Design review of the part built by this model. Coordinates are the model's own, in mm. A direction names the side the tool comes from. Round coordinates to 2 decimals unless told otherwise and drop trailing zeros. Order: outer loops, then holes, each group sorted by start corner. A loop starts at its lowest first (then second) coordinate and runs counter-clockwise, first axis right, second up. Notation, with made-up numbers: (-12, -16) - (45, -16) arc R19 cw to (45, 12) - close; hole circle Ø7 at (-38, 64.5). An arc over 180 degrees is marked (long way). Use CSV: the item, a comma, the result in double quotes. Start each with the question number.
from build123d import *

# Parameters (mm, degrees)
F0_R     = 31.75
F1_DEPTH = 50.8
F3_R     = 31.75
F4_DEPTH = 25.4
F5_W     = 63.5
F5_H     = 127
F6_DEPTH = 50.8
F7_W     = 63.5
F7_H     = 127
F8_DEPTH = 50.8


with BuildPart() as f1:
    # F0 (on Front) → F1 (new body)
    with BuildSketch(Plane.XZ):
        with BuildLine():
            ThreePointArc((0, -63.5), (44.9012806053, -44.9012806053), (63.5, 0))
            ThreePointArc((63.5, 0), (44.9012806053, 44.9012806053), (0, 63.5))
            ThreePointArc((0, 63.5), (-63.5, 0), (0, -63.5))
        make_face()
        Circle(F0_R, mode=Mode.SUBTRACT)
        with BuildLine():
            ThreePointArc((0, -63.5), (-63.5, 0), (0, 63.5))
            Line((0, 63.5), (-127, 63.5))
            Line((-127, 63.5), (-127, -63.5))
            Line((-127, -63.5), (0, -63.5))
        make_face()
    extrude(amount=F1_DEPTH)



with BuildPart() as f4:
    # F3 (on offset) → F4 (new body)
    with BuildSketch(Plane.XZ.offset(101.6)):
        with BuildLine():
            Line((-127, 63.5), (-127, -63.5))
            Line((-127, -63.5), (0, -63.5))
            ThreePointArc((0, -63.5), (63.5, 0), (0, 63.5))
            Line((0, 63.5), (-127, 63.5))
        make_face()
        Circle(F3_R, mode=Mode.SUBTRACT)
    extrude(amount=F4_DEPTH)


with BuildPart() as f6:
    # F5 (on face) → F6 (new body, through all)
    with BuildSketch(Plane.XZ.offset(50.8)):
        with Locations((-95.25, 0)):
            Rectangle(F5_W, F5_H)
    extrude(amount=F6_DEPTH)


with BuildPart() as f1_1:
    add(f1.part)

    add(f4.part)  # F8 merges F4

    add(f6.part)  # F8 merges F6
    # F7 (on face) → F8 (join, through all)
    with BuildSketch(Plane.XZ.offset(50.8)):
        with Locations((-95.25, 0)):
            Rectangle(F7_W, F7_H)
    extrude(amount=F8_DEPTH)


solid = f1_1.part
Q1. Tool access review of faces 1 (the flat face through (-29, -50.8, 15)), 2 (the flat face through (-54, 0, 1)): name each direction out of +Z, -Z, +X, -X, +Y, -Y from which nothing blocks a thin tool from reaching the whole face with its end or side.
Q2. Clearance check with flat-ended pins moving along their axes: pin 1 (2 mm diameter, centred on x = -53.5, z = -17.5, fed in from +Y); pin 2 (4 mm diameter, centred on y = -86.5, z = 9, fed in from +X). State where each tip first meets the part, or that it passes through.
Q3. Take a section at B-B (z = -15.5). State the section outline as (x, y) points, plus the area to 3 significant figures.
Q4. Take a section at D-D (y = -62.5). State the section outline as (x, z) points.
Q5. Take a section at A-A (x = -37.5). State the section outline as (y, z) points.
Q6. The part is to be moulded in two halves that separate along Z. For faces 3 (the cylindrical face through (63.485, -114.122, -1.396)), 4 (the cylindrical face through (-6.883, -25.044, -30.995)), 5 (the flat face through (-63.5, -76, -1)), say which applies: +Z half, -Z half, draft (parallel to the pull), parting line (faces both ways), or undercut.
Q7. For L1, parallel to Y at x = -16.5, z = 43; L2, parallel to Z at x = 0, y = -31; L3, parallel to X at y = -38, z = 0.5, list the stretches that pass through material, from the lowest coordinate up. Write a range as [from, to].
Q8. Take a section at C-C (y = -43). State the section outline as (x, z) points, plus the area to 3 significant figures.
Findings below:
1,face 1,"+Z, -Z, +X"
1,face 2,"+Z, -Z, +X, -X, +Y"
2,pin 1,"stops at y = 0"
2,pin 2,"stops at x = -63.5"
3,outline,"(-127, -127) - (-27.71, -127) - (-27.71, -101.6) - (-63.5, -101.6) - (-63.5, -50.8) - (-27.71, -50.8) - (-27.71, 0) - (-127, 0) - close; (27.71, -127) - (61.58, -127) - (61.58, -101.6) - (27.71, -101.6) - close; (27.71, -50.8) - (61.58, -50.8) - (61.58, 0) - (27.71, 0) - close"
3,area,"13,400 mm^2"
4,outline,"(-127, -63.5) - (-63.5, -63.5) - (-63.5, 63.5) - (-127, 63.5) - close"
5,outline,"(-127, -63.5) - (-101.6, -63.5) - (-101.6, 63.5) - (-127, 63.5) - close; (-50.8, -63.5) - (0, -63.5) - (0, 63.5) - (-50.8, 63.5) - close"
6,face 3,"parting line"
6,face 4,"undercut"
6,face 5,"draft"
7,L1,"y = [-127, -101.6], [-50.8, 0]"
7,L2,"z = [-63.5, -31.75], [31.75, 63.5]"
7,L3,"x = [-127, -31.75], [31.75, 63.5]"
8,outline,"(-127, -63.5) - (0, -63.5) arc R63.5 ccw to (0, 63.5) - (-127, 63.5) - close; hole circle Ø63.5 at (0, 0)"
8,area,"19,300 mm^2"
